from build123d import *
from build123d.topology import SkipClean

# Parameters (mm, degrees)
SKETCH1_R               = 1.65
SKETCH1_R_2             = 11
BOSS_EXTRUDE1_DEPTH     = 2
SHELL2_T                = -1
SKETCH3_R               = 4.65
SKETCH3_R_2             = 2.65
SKETCH3_R_3             = 14
SKETCH3_R_4             = 12
BOSS_EXTRUDE2_DEPTH     = 1
SKETCH4_R               = 4.65
BOSS_EXTRUDE3_DEPTH     = 1
CUT_EXTRUDE2_DEPTH      = 107.931442211
CUT_EXTRUDE2_DEPTH_BACK = 107.931442211
FILLET2_DEPTH           = 2
SKETCH7_R               = 1.65
CUT_EXTRUDE3_DEPTH      = 107.945468971
SKETCH8_R               = 3
SKETCH8_R_2             = 1.65
BOSS_EXTRUDE4_DEPTH     = 2


with BuildPart() as part:
    # Sketch1 → Boss-Extrude1 (new body)
    with BuildSketch(Plane.XY):
        Polygon((70, 40.414518843), (-70, 40.414518843), (0, -80.829037687), align=None)
        with Locations((-15.5, -15.5)):
            Circle(SKETCH1_R, mode=Mode.SUBTRACT)
        with Locations((15.5, -15.5)):
            Circle(SKETCH1_R, mode=Mode.SUBTRACT)
        with Locations((15.5, 15.5)):
            Circle(SKETCH1_R, mode=Mode.SUBTRACT)
        with Locations((-15.5, 15.5)):
            Circle(SKETCH1_R, mode=Mode.SUBTRACT)
        Circle(SKETCH1_R_2, mode=Mode.SUBTRACT)
    extrude(amount=BOSS_EXTRUDE1_DEPTH)

    # Shell2
    shell2_openings = [part.faces().sort_by_distance(p)[0] for p in [
        (0, 38.562492926, 2),
    ]]
    offset(amount=SHELL2_T, openings=shell2_openings, kind=Kind.INTERSECTION)

    # Sketch3 → Boss-Extrude2 (add)
    # profile 1 of 6: a face of its own
    with BuildSketch(Plane.XY.offset(1)):
        Polygon((68.267949192, 39.414518843), (-68.267949192, 39.414518843), (0, -78.829037687), align=None)
        Polygon((61.339745962, 35.414518843), (-61.339745962, 35.414518843), (0, -70.829037687), align=None, mode=Mode.SUBTRACT)
    # profile 2 of 6: a face of its own
    with BuildSketch(Plane.XY.offset(1)):
        with Locations((-15.5, -15.5)):
            Circle(SKETCH3_R)
        with Locations((-15.5, -15.5)):
            Circle(SKETCH3_R_2, mode=Mode.SUBTRACT)
    # profile 3 of 6: a face of its own
    with BuildSketch(Plane.XY.offset(1)):
        with Locations((15.5, -15.5)):
            Circle(SKETCH3_R)
        with Locations((15.5, -15.5)):
            Circle(SKETCH3_R_2, mode=Mode.SUBTRACT)
    # profile 4 of 6: a face of its own
    with BuildSketch(Plane.XY.offset(1)):
        Circle(SKETCH3_R_3)
        Circle(SKETCH3_R_4, mode=Mode.SUBTRACT)
    # profile 5 of 6: a face of its own
    with BuildSketch(Plane.XY.offset(1)):
        with Locations((15.5, 15.5)):
            Circle(SKETCH3_R)
        with Locations((15.5, 15.5)):
            Circle(SKETCH3_R_2, mode=Mode.SUBTRACT)
    # profile 6 of 6: a face of its own
    with BuildSketch(Plane.XY.offset(1)):
        with Locations((-15.5, 15.5)):
            Circle(SKETCH3_R)
        with Locations((-15.5, 15.5)):
            Circle(SKETCH3_R_2, mode=Mode.SUBTRACT)
    extrude(amount=BOSS_EXTRUDE2_DEPTH)

    # Sketch4 → Boss-Extrude3 (add)
    # profile 1 of 4: a face of its own
    with BuildSketch(Plane.XY.offset(1)):
        with BuildLine():
            Line((-23.337036668, -30.40810448), (-5.711087099, -12.78215491))
            ThreePointArc((-5.711087099, -12.78215491), (-9.899494937, -9.899494937), (-12.78215491, -5.711087099))
            Line((-12.78215491, -5.711087099), (-28.51341757, -21.442349758))
            Line((-28.51341757, -21.442349758), (-23.337036668, -30.40810448))
        make_face()
        with Locations((-15.5, -15.5)):
            Circle(SKETCH4_R, mode=Mode.SUBTRACT)
    # profile 2 of 4: a face of its own
    with BuildSketch(Plane.XY.offset(1)):
        with BuildLine():
            ThreePointArc((12.78215491, -5.711087099), (9.899494937, -9.899494937), (5.711087099, -12.78215491))
            Line((5.711087099, -12.78215491), (23.337036668, -30.40810448))
            Line((23.337036668, -30.40810448), (28.51341757, -21.442349758))
            Line((28.51341757, -21.442349758), (12.78215491, -5.711087099))
        make_face()
        with Locations((15.5, -15.5)):
            Circle(SKETCH4_R, mode=Mode.SUBTRACT)
    # profile 3 of 4: a face of its own
    with BuildSketch(Plane.XY.offset(1)):
        with BuildLine():
            ThreePointArc((5.711087099, 12.78215491), (9.899494937, 9.899494937), (12.78215491, 5.711087099))
            Line((12.78215491, 5.711087099), (42.485586655, 35.414518843))
            Line((42.485586655, 35.414518843), (28.343451031, 35.414518843))
            Line((28.343451031, 35.414518843), (5.711087099, 12.78215491))
        make_face()
        with Locations((15.5, 15.5)):
            Circle(SKETCH4_R, mode=Mode.SUBTRACT)
    # profile 4 of 4: a face of its own
    with BuildSketch(Plane.XY.offset(1)):
        with BuildLine():
            Line((-42.485586655, 35.414518843), (-12.78215491, 5.711087099))
            ThreePointArc((-12.78215491, 5.711087099), (-9.899494937, 9.899494937), (-5.711087099, 12.78215491))
            Line((-5.711087099, 12.78215491), (-28.343451031, 35.414518843))
            Line((-28.343451031, 35.414518843), (-42.485586655, 35.414518843))
        make_face()
        with Locations((-15.5, 15.5)):
            Circle(SKETCH4_R, mode=Mode.SUBTRACT)
    extrude(amount=BOSS_EXTRUDE3_DEPTH)

    # Sketch6 → Cut-Extrude2 (cut, two sides: drawn at the far end of the back side and taken through both)
    with BuildSketch(Plane.XY.offset(1).offset(-CUT_EXTRUDE2_DEPTH_BACK)):
        with BuildLine():
            Line((-12.78215491, 5.711087099), (-42.485586655, 35.414518843))
            Line((-42.485586655, 35.414518843), (-61.339745962, 35.414518843))
            Line((-61.339745962, 35.414518843), (-28.51341757, -21.442349758))
            Line((-28.51341757, -21.442349758), (-12.78215491, -5.711087099))
            ThreePointArc((-12.78215491, -5.711087099), (-14, 0), (-12.78215491, 5.711087099))
        make_face()
        with BuildLine():
            Line((0, -70.829037687), (23.337036668, -30.40810448))
            Line((23.337036668, -30.40810448), (5.711087099, -12.78215491))
            ThreePointArc((5.711087099, -12.78215491), (0, -14), (-5.711087099, -12.78215491))
            Line((-5.711087099, -12.78215491), (-23.337036668, -30.40810448))
            Line((-23.337036668, -30.40810448), (0, -70.829037687))
        make_face()
        with BuildLine():
            Line((42.485586655, 35.414518843), (12.78215491, 5.711087099))
            ThreePointArc((12.78215491, 5.711087099), (14, 0), (12.78215491, -5.711087099))
            Line((12.78215491, -5.711087099), (28.51341757, -21.442349758))
            Line((28.51341757, -21.442349758), (61.339745962, 35.414518843))
            Line((61.339745962, 35.414518843), (42.485586655, 35.414518843))
        make_face()
        with BuildLine():
            Line((-28.343451031, 35.414518843), (-5.711087099, 12.78215491))
            ThreePointArc((-5.711087099, 12.78215491), (0, 14), (5.711087099, 12.78215491))
            Line((5.711087099, 12.78215491), (28.343451031, 35.414518843))
            Line((28.343451031, 35.414518843), (-28.343451031, 35.414518843))
        make_face()
    extrude(amount=CUT_EXTRUDE2_DEPTH + CUT_EXTRUDE2_DEPTH_BACK, mode=Mode.SUBTRACT)

    # Fillet2: read off the stored shape, not the designer's step
    # Fillet2 outline → Fillet2 (add)
    with SkipClean():  # the faces are left unmerged after this step: merging them gives an invalid solid
        with BuildSketch(Plane.XY):
            with BuildLine():
                ThreePointArc((4.330127019, -63.329037687), (0, -65.829037687), (-4.330127019, -63.329037687))
                Line((-4.330127019, -63.329037687), (0, -70.829037687))
                Line((0, -70.829037687), (4.330127019, -63.329037687))
            make_face()
            with BuildLine():
                ThreePointArc((52.679491924, 35.414518843), (57.009618943, 32.914518843), (57.009618943, 27.914518843))
                Line((57.009618943, 27.914518843), (61.339745962, 35.414518843))
                Line((61.339745962, 35.414518843), (52.679491924, 35.414518843))
            make_face()
            with BuildLine():
                ThreePointArc((-57.009618943, 27.914518843), (-57.009618943, 32.914518843), (-52.679491924, 35.414518843))
                Line((-52.679491924, 35.414518843), (-61.339745962, 35.414518843))
                Line((-61.339745962, 35.414518843), (-57.009618943, 27.914518843))
            make_face()
        extrude(amount=FILLET2_DEPTH)
    add(part.part.scale(1), mode=Mode.REPLACE)  # the faces are merged on a copy

    # Sketch7 → Cut-Extrude3 (cut, through all)
    with BuildSketch(Plane.XY.offset(2)):
        with Locations((-62.5, 36.084391824)):
            Circle(SKETCH7_R)
        with Locations((62.5, 36.084391824)):
            Circle(SKETCH7_R)
        with Locations((0, -72.168783649)):
            Circle(SKETCH7_R)
    extrude(amount=-CUT_EXTRUDE3_DEPTH, mode=Mode.SUBTRACT)

    # Sketch8 → Boss-Extrude4 (add)
    # profile 1 of 4: a face of its own
    with BuildSketch(Plane.XY.offset(2)):
        with Locations((-15.5, 15.5)):
            Circle(SKETCH8_R)
        with Locations((-15.5, 15.5)):
            Circle(SKETCH8_R_2, mode=Mode.SUBTRACT)
    # profile 2 of 4: a face of its own
    with BuildSketch(Plane.XY.offset(2)):
        with Locations((15.5, 15.5)):
            Circle(SKETCH8_R)
        with Locations((15.5, 15.5)):
            Circle(SKETCH8_R_2, mode=Mode.SUBTRACT)
    # profile 3 of 4: a face of its own
    with BuildSketch(Plane.XY.offset(2)):
        with Locations((15.5, -15.5)):
            Circle(SKETCH8_R)
        with Locations((15.5, -15.5)):
            Circle(SKETCH8_R_2, mode=Mode.SUBTRACT)
    # profile 4 of 4: a face of its own
    with BuildSketch(Plane.XY.offset(2)):
        with Locations((-15.5, -15.5)):
            Circle(SKETCH8_R)
        with Locations((-15.5, -15.5)):
            Circle(SKETCH8_R_2, mode=Mode.SUBTRACT)
    extrude(amount=BOSS_EXTRUDE4_DEPTH)


solid = part.part
Source: CAD feature listing. Evaluate the final solid. Frame: model axes, mm. A direction names the side the tool comes from. Round coordinates to 2 decimals unless told otherwise and drop trailing zeros. Loops run counter-clockwise (first coordinate to the right, second up) from the corner with the lowest first, then second, coordinate; pieces in that order, holes last.
Q1. Access query for faces 1 (the face through (-14, -17, 4)), 2 (the face through (-16.15, 12.57, 2.99)), 3 (the face through (-57.046, 32.851, 0.986)). Directions: +Z, -Z, +X, -X, +Y, -Y. A direction counts if a zero-diameter tool reaches every point of the face in a straight line with its end or side. Return the directions, or none.
Q2. Mould query, pull axis X, two halves, no side actions, for faces 4 (the face through (13.1, -17.3, 3)), 5 (the face through (34.51, -21.056, 0.986)), 6 (the face through (60.85, 36.16, 1.01)), 7 (the face through (17, -17, 4)). Classes: pulls with the +X half, pulls with the -X half, needs draft (parallel to the pull), parting line crosses it, or undercut.
Q3. First-contact query: P1, Ø2.5, axis at x = -15.5, y = 15.5, coming from the +Z side; P2, Ø2, axis at x = 32, z = 2.5, coming from the -Y side; P3, Ø1.1, axis at x = 6.5, z = 0.5, coming from the -Y side; P4, Ø4.5, axis at x = 15.5, y = -15.5, coming from the -Z side. Flat tips, straight axial feed; report the tip coordinate or a pass-through.
Q4. Section C-C, the plane y = 15.5. State how many separate pieces and enclosed holes the cut face has, plus the area to 3 significant figures.
Q5. Section A-A, the plane z = 2.6. Return loops of the section in (x, y).
Q6. Section B-B, the plane x = 35.5. Return loops of the section in (y, z), plus the area to 3 significant figures.
Q7. Ray query, line 1 (Y direction, x = 0, z = 0.65); line 2 (Y direction, x = 15.5, z = 2.95); line 3 (Y direction, x = 3, z = 1.2). Return the intervals inside material, ascending.
Solutions:
1. face 1: +Z, +X, -X, +Y, -Y
1. face 2: +Z
1. face 3: +Z, -Z
2. face 4: undercut
2. face 5: pulls with the +X half
2. face 6: undercut
2. face 7: needs draft
3. P1: passes through
3. P2: stops at y = -26.9
3. P3: stops at y = -70.52
3. P4: stops at z = 0
4. separate pieces: 6
4. enclosed holes: 0
4. area: 77.3 mm2
5. outline: circle Ø6 at (-15.5, -15.5); circle Ø6 at (-15.5, 15.5); circle Ø6 at (15.5, -15.5); circle Ø6 at (15.5, 15.5); hole circle Ø3.3 at (-15.5, -15.5); hole circle Ø3.3 at (-15.5, 15.5); hole circle Ø3.3 at (15.5, -15.5); hole circle Ø3.3 at (15.5, 15.5)
6. outline: (-19.34, 0) - (-9.34, 0) - (-9.34, 2) - (-19.34, 2) - close; (28.43, 0) - (40.41, 0) - (40.41, 2) - (28.43, 2) - close
6. area: 44.0 mm2
7. line 1: y = -80.83 to -73.82, -70.52 to -65.83, -14 to -11, 11 to 14, 35.41 to 40.41
7. line 2: y = -18.5 to -17.15, -13.85 to -12.5, 12.5 to 13.85, 17.15 to 18.5
7. line 3: y = -75.63 to -64.83, -13.67 to -10.58, 10.58 to 13.67, 35.41 to 40.41
